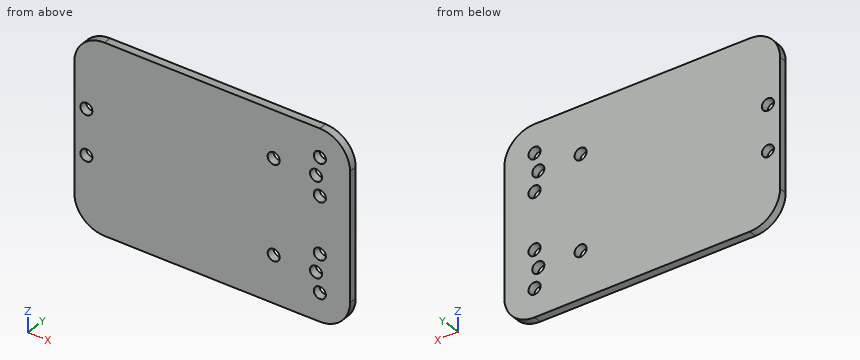
```python
from build123d import *

# Parameters (mm, degrees)
SKETCH_1_W          = 73
SKETCH_1_H          = 50
EXTRUDE_1_DEPTH     = 2.1
SKETCH_2_R          = 1.6
CUT_EXTRUDE_1_DEPTH = 2.1
SKETCH_3_R          = 1.6
CUT_EXTRUDE_2_DEPTH = 2.1
SKETCH_4_R          = 1.6
CUT_EXTRUDE_3_DEPTH = 2.1
FILLET_1_R          = 8


with BuildPart() as part:
    # 草图1 → 凸台-拉伸1 (new body)
    with BuildSketch(Plane(origin=(0, 0, 0), x_dir=(1, 0, 0), z_dir=(0, 1, 0))):
        Rectangle(SKETCH_1_W, SKETCH_1_H)
    extrude(amount=EXTRUDE_1_DEPTH)

    # 草图2 → 切除-拉伸1 (cut)
    with BuildSketch(Plane(origin=(0, 2.1, 0), x_dir=(1, 0, 0), z_dir=(0, 1, 0))):
        with Locations(Location((-33.3, 6, 0), (0, 0, 270))):
            Circle(SKETCH_2_R)
        with Locations(Location((-33.3, -6, 0), (0, 0, 270))):
            Circle(SKETCH_2_R)
    extrude(amount=-CUT_EXTRUDE_1_DEPTH, mode=Mode.SUBTRACT)

    # 草图3 → 切除-拉伸2 (cut)
    with BuildSketch(Plane(origin=(0, 2.1, 0), x_dir=(1, 0, 0), z_dir=(0, 1, 0))):
        with Locations(Location((28.5, 17.5, 0), (0, 0, 270))):
            Circle(SKETCH_3_R)
        with Locations(Location((28.5, 7.5, 0), (0, 0, 270))):
            Circle(SKETCH_3_R)
        with Locations(Location((28.5, -7.5, 0), (0, 0, 270))):
            Circle(SKETCH_3_R)
        with Locations(Location((28.5, -17.5, 0), (0, 0, 270))):
            Circle(SKETCH_3_R)
    extrude(amount=-CUT_EXTRUDE_2_DEPTH, mode=Mode.SUBTRACT)

    # 草图4 → 切除-拉伸3 (cut)
    with BuildSketch(Plane(origin=(0, 2.1, 0), x_dir=(1, 0, 0), z_dir=(0, 1, 0))):
        with Locations(Location((16.3, 12.5, 0), (0, 0, 270))):
            Circle(SKETCH_4_R)
        with Locations(Location((16.3, -12.5, 0), (0, 0, 270))):
            Circle(SKETCH_4_R)
        with Locations(Location((27.5, 12.5, 0), (0, 0, 270))):
            Circle(SKETCH_4_R)
        with Locations(Location((27.5, -12.5, 0), (0, 0, 270))):
            Circle(SKETCH_4_R)
    extrude(amount=-CUT_EXTRUDE_3_DEPTH, mode=Mode.SUBTRACT)

    # 圆角1
    fillet_1_edges = [part.edges().sort_by_distance(p)[0] for p in [
        (36.5, 1.05, 25),
        (-36.5, 1.05, 25),
        (-36.5, 1.05, -25),
        (36.5, 1.05, -25),
    ]]
    fillet(fillet_1_edges, radius=FILLET_1_R)


solid = part.part
```
Could you check a few things on this model? Use its own coordinates, in mm. Coordinates: 2 decimals unless noted, no trailing zeros. Loops run counter-clockwise (first coordinate to the right, second up) from the corner with the lowest first, then second, coordinate; pieces in that order, holes last. Notation, with made-up numbers: M 86,85.25 L 130,85.25 A13 cw 130,100.25 Z; hole C 40,56.5 d3. An arc over 180 degrees is marked long. Put each result on its own line as item: value. Start each with the question number.
(1) Suppose I cut it at C-C on y = 1.45. Count the separate pieces of the cut face and the enclosed holes in it, then the cut area to 3 significant figures.
(2) I need wall thicknesses on line 1 (X direction, y = 1.35, z = 12.5); line 2 (X direction, y = 1, z = 17.5); line 3 (Z direction, x = 17.5, y = 0.75). Which ranges of each line are inside material? Lowest first, please. Write a range as from..to.
(3) Suppose I cut it at B-B on x = 16.3. Please give me the cut outline in (y, z), then the cut area to 3 significant figures.
(4) Suppose I cut it at A-A on z = -12.5. Please give me the cut outline in (x, y), then the cut area to 3 significant figures.
Solutions:
1. separate pieces: 1
1. enclosed holes: 10
1. area: 3,510 mm2
2. line 1: x = -36.5..14.7, 17.9..25.9, 29.1..36.5
2. line 2: x = -36.48..26.9, 30.1..36.48
2. line 3: z = -25..-13.56, -11.44..11.44, 13.56..25
3. outline: M 0,-25 L 2.1,-25 L 2.1,-14.1 L 0,-14.1 Z; M 0,-10.9 L 2.1,-10.9 L 2.1,10.9 L 0,10.9 Z; M 0,14.1 L 2.1,14.1 L 2.1,25 L 0,25 Z
3. area: 91.6 mm2
4. outline: M -36.5,0 L 14.7,0 L 14.7,2.1 L -36.5,2.1 Z; M 17.9,0 L 25.9,0 L 25.9,2.1 L 17.9,2.1 Z; M 29.1,0 L 36.5,0 L 36.5,2.1 L 29.1,2.1 Z
4. area: 140 mm2
